Can you work these out from the model? Positions are in its coordinate system, mm. Face numbers are marked on the shaded views. A direction names the side the tool comes from. Round coordinates to 2 decimals unless told otherwise and drop trailing zeros. Order: outer loops, then holes, each group sorted by start corner. A loop starts at its lowest first (then second) coordinate and runs counter-clockwise, first axis right, second up.
Q1. For the marked faces 1, 2 and 3, which set-ups out of +Z, -Z, +X, -X, +Y, -Y let a thin tool reach every point of the face, with its end or its side?
Q2. We'd pull the mould along Y, two halves only. Please class the marked faces 4, 5 and 6: pulls with the +Y half, pulls with the -Y half, needs draft (parallel to the pull), parting line crosses it, or undercut.
Q3. If we section it at C-C (x = 848): Please give me the cut outline in (y, z).
Q4. If we section it at A-A (y = 0): Count the separate pieces of the cut face and the enclosed holes in it, plus the area to 3 significant figures.
Q5. If we section it at D-D (x = 165): Please give me the cut outline in (y, z), plus the area to 3 significant figures.
Q6. Will these pins go through, and if not, where does the flat tip stop? P1, Ø6, axis at y = 67, z = 51, coming from the +X side; P2, Ø1, axis at y = -66.5, z = 19, coming from the -X side; P3, Ø14, axis at y = -56, z = 0, coming from the -X side.
Q7. If I drill on line 1 (Y direction, x = 673, z = 30.5); line 2 (Y direction, x = 206, z = 0); line 3 (X direction, y = 30, z = -70), over which ranges is the centre line in solid material (lowest first)?
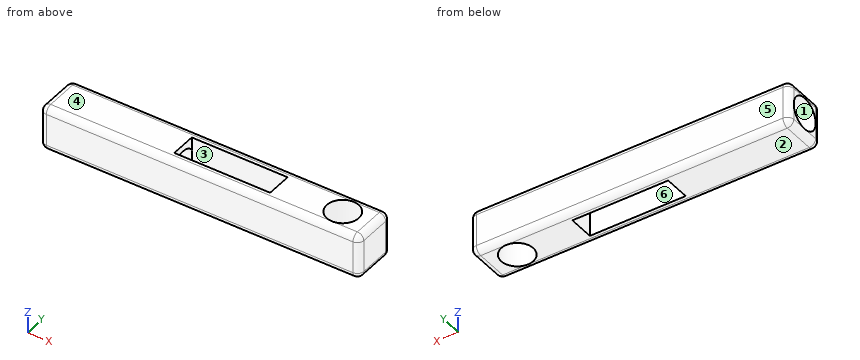
from build123d import *

# Parameters (mm, degrees)
F0_W     = 177.8
F0_H     = 177.8
F1_DEPTH = 1270
F2_R     = 63.5
F3_DEPTH = 177.8
F4_R     = 63.5
F5_DEPTH = 508
F6_R     = 25.4
F7_R     = 25.4
F8_W     = 381
F8_H     = 101.6
F9_DEPTH = 177.8
F10_R    = 25.39999


# Not quite as in the source:
# - a fillet or chamfer is up to 0.001 mm smaller than in the source, because OpenCascade refuses the exact size


with BuildPart() as f1:
    # F0 (on Right) → F1 (new body)
    with BuildSketch(Plane.YZ):
        Rectangle(F0_W, F0_H)
    extrude(amount=F1_DEPTH)

    # F2 (on face) → F3 (cut)
    with BuildSketch(Plane.XY.offset(88.9)):
        with Locations((1143, 0)):
            Circle(F2_R)
    extrude(amount=-F3_DEPTH, mode=Mode.SUBTRACT)

    # F4 (on face) → F5 (cut)
    with BuildSketch(Plane(origin=(0, 0, 0), x_dir=(0, -1, 0), z_dir=(-1, 0, 0))):
        Circle(F4_R)
    extrude(amount=-F5_DEPTH, mode=Mode.SUBTRACT)

    # F6
    f6_edges = [f1.edges().sort_by_distance(p)[0] for p in [
        (635, -88.9, 88.9),
        (635, 88.9, 88.9),
        (635, -88.9, -88.9),
        (635, 88.9, -88.9),
    ]]
    fillet(f6_edges, radius=F6_R)

    # F7
    f7_edges = [f1.edges().sort_by_distance(p)[0] for p in [
        (1270, 0, 88.9),
    ]]
    fillet(f7_edges, radius=F7_R)

    # F8 (on face) → F9 (cut)
    with BuildSketch(Plane.XY.offset(88.9)):
        with Locations((698.5, 0)):
            Rectangle(F8_W, F8_H)
    extrude(amount=-F9_DEPTH, mode=Mode.SUBTRACT)

    # F10 (radius 25.4 in the source; OpenCascade refuses exactly that, so slightly less here)
    f10_edges = [f1.edges().sort_by_distance(p)[0] for p in [
        (0, 0, 88.9),
    ]]
    fillet(f10_edges, radius=F10_R)


solid = f1.part
Solution:
1. face 1: -X
1. face 2: -Z, +X, -X, +Y, -Y
1. face 3: +Z, -Z
2. face 4: needs draft
2. face 5: pulls with the +Y half
2. face 6: undercut
3. outline: (-88.9, -63.5) arc R25.4 ccw to (-63.5, -88.9) - (-50.8, -88.9) - (-50.8, 88.9) - (-63.5, 88.9) arc R25.4 ccw to (-88.9, 63.5) - close; (50.8, -88.9) - (63.5, -88.9) arc R25.4 ccw to (88.9, -63.5) - (88.9, 63.5) arc R25.4 ccw to (63.5, 88.9) - (50.8, 88.9) - close
4. separate pieces: 4
4. enclosed holes: 0
4. area: 70,400 mm2
5. outline: (-88.9, -63.5) arc R25.4 ccw to (-63.5, -88.9) - (63.5, -88.9) arc R25.4 ccw to (88.9, -63.5) - (88.9, 63.5) arc R25.4 ccw to (63.5, 88.9) - (-63.5, 88.9) arc R25.4 ccw to (-88.9, 63.5) - close; hole circle Ø127 at (0, 0)
5. area: 18,400 mm2
6. P1: stops at x = 1270
6. P2: stops at x = 0.12
6. P3: stops at x = 508
7. line 1: y = -88.9 to -50.8, 50.8 to 88.9
7. line 2: y = -88.9 to -63.5, 63.5 to 88.9
7. line 3: x = 0.85 to 508, 889 to 1087.03, 1198.97 to 1269.15
